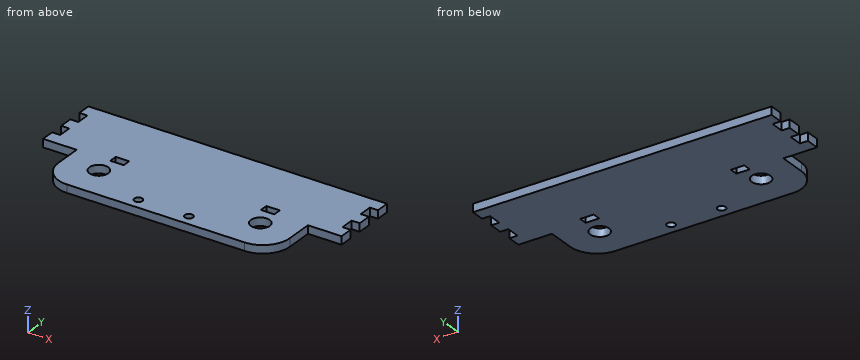
Autodesk Inventor part; units mm, degrees
ref_plane "YZ Plane" through (0, 0, 0) normal (1, 0, 0) x (0, 1, 0)
ref_plane "XZ Plane" through (0, 0, 0) normal (0, 1, 0) x (-1, 0, 0)
ref_plane "XY Plane" through (0, 0, 0) normal (0, 0, 1) x (1, 0, 0)
sketch "Sketch1" plane through (0, 0, 0) normal (0, 0, 1) x (1, 0, 0)
  line L0 (12.5, 0) -> (98.5, 0)
  line L1 (111, 45) -> (0, 45)
  line L2 (12.5, 20) -> (12.5, 0)
  line L3 (111, 20) -> (98.5, 20) construction
  line L4 (111, 20) -> (98.5, 20)
  line L5 (98.5, 20) -> (98.5, 0)
  line L6 (12.5, 20) -> (0, 20)
  line L7 (12.5, 0) -> (25.5, 0) construction
  line L8 (12.5, 13) -> (12.5, 0) construction
  line L9 (98.5, 0) -> (85.5, 0) construction
  line L10 (98.5, 13) -> (98.5, 0) construction
  line L11 (0, 45) -> (0, 40)
  line L12 (0, 40) -> (3, 40)
  line L13 (3, 40) -> (3, 35)
  line L14 (3, 35) -> (0, 35)
  line L15 (0, 35) -> (0, 30)
  line L16 (0, 30) -> (3, 30)
  line L17 (3, 30) -> (3, 25)
  line L18 (3, 25) -> (0, 25)
  line L19 (0, 25) -> (0, 20)
  line L20 (0, 45) -> (0, 40)
  line L21 (0, 35) -> (0, 30)
  line L22 (0, 25) -> (0, 20)
  line L23 (111, 45) -> (111, 40)
  line L24 (111, 40) -> (108, 40)
  line L25 (108, 40) -> (108, 35)
  line L26 (108, 35) -> (111, 35)
  line L27 (111, 35) -> (111, 30)
  line L28 (111, 30) -> (108, 30)
  line L29 (108, 30) -> (108, 25)
  line L30 (108, 25) -> (111, 25)
  line L31 (111, 25) -> (111, 20)
  line L32 (111, 40) -> (111, 45)
  line L33 (111, 20) -> (111, 25)
  line L34 (111, 30) -> (111, 35)
  circle A0 centre (25.5, 13) radius 3.5
  circle A1 centre (85.5, 13) radius 3.5
  dimension "d52" = 7
  dimension "d53" = 7
extrude "Extrusion1" add sketch "Sketch1" against normal blind 3 contours L2 L6 L19 L18 L17 L16 L15 L14 L13 L12 L11 L1 L23 L24 L25 L26 L27 L28 L29 L30 L31 L4 L5 L0 | A0 | A1
fillet "Fillet1" radius 10 2 edges at (12.5, 0, -1.5) (98.5, 0, -1.5)
sketch "Sketch2" plane through (0, 0, 0) normal (0, 0, 1) x (1, 0, 0)
  line L0 (25, 20) -> (30, 20)
  line L1 (30, 20) -> (30, 23)
  line L2 (30, 23) -> (25, 23)
  line L3 (25, 23) -> (25, 20)
  line L4 (86, 20) -> (81, 20)
  line L5 (81, 20) -> (81, 23)
  line L6 (81, 23) -> (86, 23)
  line L7 (86, 23) -> (86, 20)
  point P0 (0, 0)
  point P1 (0, 20)
  point P2 (111, 20)
  dimension "d32" = 5
  dimension "d33" = 3
  dimension "d34" = 5
  dimension "d35" = 25
  dimension "d36" = 5
  dimension "d37" = 3
  dimension "d38" = 5
extrude "Extrusion3" cut sketch "Sketch2" against normal blind 10
sketch "Sketch3" plane through (0, 0, 0) normal (0, 0, 1) x (1, 0, 0)
  circle A0 centre (64.9, 4.25) radius 1.5
  line L0 (0, 45) -> (111, 45)
  circle A1 centre (46.1, 4.25) radius 1.5
  point P0 (0, 0)
  point P1 (85.5, 13)
  dimension "d49" = 3
  dimension "d50" = 3
extrude "Extrusion4" cut sketch "Sketch3" against normal blind 10
extrude "Extrusion5" cut sketch "Sketch1" against normal blind 10 contours A0 | A1
properties part number "Zijkant"
Geometry check sheet. Reference: the model listing, model coordinates, mm. Round coordinates to 2 decimals unless told otherwise and drop trailing zeros. Order: outer loops, then holes, each group sorted by start corner. A loop starts at its lowest first (then second) coordinate and runs counter-clockwise, first axis right, second up. Notation, with made-up numbers: (36.25, 82.5) - (95.25, 82.5) arc R31 cw to (95.25, 107.5) - close; hole circle Ø4 at (1, 23). An arc over 180 degrees is marked (long way). Use a Markdown table: item, result. Add a question column.
(1) Sectioned sample at A-A, the plane y = 13. Enter the section's corners in (x, z).
(2) Depth check by flat-ended pin: pin 1 (1.5 mm diameter, centred on x = 1.5, z = -1.5, fed in from -Y); pin 2 (0.9 mm diameter, centred on y = 16, z = -1.5, fed in from +X). Enter the tip coordinate at first touch or a pass-through.
(3) Sectioned sample at D-D, the plane y = 4.25. Enter the section's corners in (x, z).
(4) Sectioned sample at B-B, the plane x = 46.1. Enter the section's corners in (y, z), and give its area (3 significant figures).
(5) Material ranges on line 1 along Y through (x, z) = (85.5, -1.35); line 2 along X through (y, z) = (21.5, -1.2); line 3 along Y through (x, z) = (64.9, -0.7), recorded low to high. Write a range as [from, to].
(6) Sectioned sample at C-C, the plane z = -1.8. Count the separate pieces of the cut face and the enclosed holes in it, and give its area (3 significant figures).
Answers below:
| question | item | result |
|---|---|---|
| 1 | outline | (12.5, -3) - (22, -3) - (22, 0) - (12.5, 0) - close; (29, -3) - (82, -3) - (82, 0) - (29, 0) - close; (89, -3) - (98.5, -3) - (98.5, 0) - (89, 0) - close |
| 2 | pin 1 | y = 20 |
| 2 | pin 2 | x = 98.5 |
| 3 | outline | (14.32, -3) - (44.6, -3) - (44.6, 0) - (14.32, 0) - close; (47.6, -3) - (63.4, -3) - (63.4, 0) - (47.6, 0) - close; (66.4, -3) - (96.68, -3) - (96.68, 0) - (66.4, 0) - close |
| 4 | outline | (0, -3) - (2.75, -3) - (2.75, 0) - (0, 0) - close; (5.75, -3) - (45, -3) - (45, 0) - (5.75, 0) - close |
| 4 | area | 126 mm² |
| 5 | line 1 | [0, 9.5], [16.5, 20], [23, 45] |
| 5 | line 2 | [0, 25], [30, 81], [86, 111] |
| 5 | line 3 | [0, 2.75], [5.75, 45] |
| 6 | separate pieces | 1 |
| 6 | enclosed holes | 6 |
| 6 | area | 4,270 mm² |
